Here's how the part is built. I have some questions about the finished solid (model axes, mm). A direction names the side the tool comes from. Give positions to 0.01 mm unless a question says otherwise; leave off trailing zeros. Write each loop counter-clockwise with the first axis right and the second up, starting at its lowest first coordinate (ties: lowest second). Pieces come first, ordered by that corner, then holes. Notation, with made-up numbers: (33.25, 58.25) -> (47.25, 58.25) arc R25 cw to (47.25, 88.25) -> close; hole circle Ø4 at (-34.75, 57.5). An arc over 180 degrees is marked (long way). Return JSON: item names as keys, results as strings.
from build123d import *

# Parameters (mm, degrees)
SKETCH1_W           = 19.05
SKETCH1_H           = 19.05
BOSS_EXTRUDE2_DEPTH = 6.35
SKETCH8_W           = 217.17
SKETCH8_H           = 38.1
BOSS_EXTRUDE4_DEPTH = 6.35
SKETCH8_5_W         = 217.17
SKETCH8_5_H         = 38.1
BOSS_EXTRUDE5_DEPTH = 6.4262
SKETCH9_W           = 19.05
SKETCH9_H           = 38.1
LPATTERN3_COUNT     = 11
LPATTERN3_PITCH     = 19.812
SKETCH15_R          = 12.192
BOSS_EXTRUDE6_DEPTH = 6.35
SKETCH16_W          = 38.1
SKETCH16_H          = 22.073264639
CUT_EXTRUDE1_DEPTH  = 3.302
SKETCH17_W          = 61.644203732
SKETCH17_H          = 46.422477749
CUT_EXTRUDE2_DEPTH  = 137.922
SKETCH18_W          = 24.384
SKETCH18_H          = 9.5504
BOSS_EXTRUDE7_DEPTH = 12.7


with BuildPart() as part:
    # Sketch1 → Boss-Extrude2 (new body)
    with BuildSketch(Plane(origin=(0, 0, 0), x_dir=(1, 0, 0), z_dir=(0, 1, 0))):
        with Locations((9.525, -9.525)):
            Rectangle(SKETCH1_W, SKETCH1_H)
    extrude(amount=BOSS_EXTRUDE2_DEPTH)

    # Sketch8 → Boss-Extrude4 (add)
    with BuildSketch(Plane(origin=(0, 0, 0), x_dir=(1, 0, 0), z_dir=(0, 1, 0))):
        with Locations((108.585, -9.525)):
            Rectangle(SKETCH8_W, SKETCH8_H)
    extrude(amount=BOSS_EXTRUDE4_DEPTH)

    # Sketch8<5> → Boss-Extrude5 (add)
    with BuildSketch(Plane(origin=(0, 0, 0), x_dir=(1, 0, 0), z_dir=(0, 1, 0))):
        with Locations((108.585, -9.525)):
            Rectangle(SKETCH8_5_W, SKETCH8_5_H)
    extrude(amount=-BOSS_EXTRUDE5_DEPTH)

    # Sketch9 → Loft3 section 0
    with BuildSketch(Plane(origin=(0, 6.35, 0), x_dir=(1, 0, 0), z_dir=(0, 1, 0)), mode=Mode.PRIVATE) as loft3_s0:
        with Locations((9.525, -9.525)):
            Rectangle(SKETCH9_W, SKETCH9_H)
    loft3 = loft([loft3_s0.sketch, Vertex(9.525, 26.0731, 19.05)])

    # LPattern3: Loft3 ×11
    with Locations(*[(i * LPATTERN3_PITCH, 0, 0) for i in range(1, LPATTERN3_COUNT)]):
        add(loft3)

    # Sketch15 → Boss-Extrude6 (add)
    with BuildSketch(Plane.XZ.offset(6.4262)):
        with Locations((179.07, 9.525)):
            Circle(SKETCH15_R)
        with Locations((38.1, 9.525)):
            Circle(SKETCH15_R)
        with Locations((108.585, 9.525)):
            Circle(SKETCH15_R)
    extrude(amount=BOSS_EXTRUDE6_DEPTH)

    # Sketch16 → Cut-Extrude1 (cut)
    with BuildSketch(Plane(origin=(219.71, 0, 0), x_dir=(0, 0, -1), z_dir=(1, 0, 0))):
        with Locations((-9.525, 4.61043232)):
            Rectangle(SKETCH16_W, SKETCH16_H)
    extrude(amount=-CUT_EXTRUDE1_DEPTH, mode=Mode.SUBTRACT)

    # Sketch17 → Cut-Extrude2 (cut)
    with BuildSketch(Plane.ZY):
        with Locations((9.467504242, 6.577579821)):
            Rectangle(SKETCH17_W, SKETCH17_H)
    extrude(amount=-CUT_EXTRUDE2_DEPTH, mode=Mode.SUBTRACT)

    # Sketch18 → Boss-Extrude7 (add)
    with BuildSketch(Plane.ZY.offset(-137.922)):
        with Locations((9.525, -0.0381)):
            Rectangle(SKETCH18_W, SKETCH18_H)
    extrude(amount=BOSS_EXTRUDE7_DEPTH)


solid = part.part
1. Suppose I cut it at A-A, the plane y = 10. List the corners of the cut face in (x, z) for me.
Taken from the geometry:
{"outline": "(140.45, -4.24) -> (155.97, -4.24) -> (155.97, 26.81) -> (140.45, 26.81) -> close; (160.26, -4.24) -> (175.78, -4.24) -> (175.78, 26.81) -> (160.26, 26.81) -> close; (180.07, -4.24) -> (195.6, -4.24) -> (195.6, 26.81) -> (180.07, 26.81) -> close; (199.88, -4.24) -> (215.41, -4.24) -> (215.41, 26.81) -> (199.88, 26.81) -> close"}
2. Suppose I cut it at C-C, the plane z = 3.5. List the corners of the cut face in (x, y) for me.
Taken from the geometry:
{"outline": "(125.22, -4.81) -> (137.92, -4.81) -> (137.92, -6.43) -> (168.47, -6.43) -> (168.47, -12.78) -> (189.67, -12.78) -> (189.67, -6.43) -> (216.41, -6.43) -> (216.41, 7.93) -> (212.83, 15.34) -> (202.46, 15.34) -> (198.12, 6.35) -> (197.36, 6.35) -> (193.02, 15.34) -> (182.65, 15.34) -> (178.31, 6.35) -> (177.55, 6.35) -> (173.2, 15.34) -> (162.84, 15.34) -> (158.5, 6.35) -> (157.73, 6.35) -> (153.39, 15.34) -> (143.03, 15.34) -> (138.68, 6.35) -> (137.92, 6.35) -> (137.92, 4.74) -> (125.22, 4.74) -> close"}
3. If I drill on line 1 (X direction, y = 12.5, z = 18.5); line 2 (Y direction, x = 178, z = 21); line 3 (X direction, y = 6, z = -2), over which ranges is the centre line in solid material (lowest first)? Write a range as [from, to].
Taken from the geometry:
{"line 1": "x = [141.65, 154.76], [161.47, 174.58], [181.28, 194.39], [201.09, 214.2]", "line 2": "y = [-12.78, 6.35]", "line 3": "x = [137.92, 216.41]"}
4. Suppose I cut it at B-B, the plane x = 175.5. List the corners of the cut face in (y, z) for me (3 decimals), and give its area (3 significant figures).
Taken from the geometry:
{"outline": "(-12.776, -2.133) -> (-6.426, -2.133) -> (-6.426, -9.525) -> (6.35, -9.525) -> (10.587, -3.387) -> (10.587, 26.529) -> (6.35, 28.575) -> (-6.426, 28.575) -> (-6.426, 21.183) -> (-12.776, 21.183) -> close", "area": "779 mm²"}
5. Suppose I cut it at D-D, the plane y = 23.5. List the corners of the cut face in (x, z) for me.
Taken from the geometry:
{"outline": "(146.97, 15.32) -> (149.45, 15.32) -> (149.45, 20.29) -> (146.97, 20.29) -> close; (166.78, 15.32) -> (169.26, 15.32) -> (169.26, 20.29) -> (166.78, 20.29) -> close; (186.59, 15.32) -> (189.08, 15.32) -> (189.08, 20.29) -> (186.59, 20.29) -> close; (206.4, 15.32) -> (208.89, 15.32) -> (208.89, 20.29) -> (206.4, 20.29) -> close"}
6. For pin 1 Ø4 at (x, z) = (197.5, 8.5) entering from +Y; pin 2 Ø3 at (x, z) = (201.5, -1.5) entering from -Y; pin 3 Ø5 at (y, z) = (11.5, 6) entering from +X, each with a flat end and sliding along its axis, tell me the tip position at first contact or that it passes through.
Taken from the geometry:
{"pin 1": "stops at y = 10.2", "pin 2": "stops at y = -6.43", "pin 3": "stops at x = 215.89"}
7. Which directions (+Z, -Z, +X, -X, +Y, -Y) give clear straight access to the entire face, cutting with the end or side of a thin tool? Please do faces 1 (the face through (132, 0, 21.717)), 2 (the face through (174.83, 11.97, 14.03)), 3 (the face through (132, -4.813, 9)).
Taken from the geometry:
{"face 1": "+Z, -X, +Y, -Y", "face 2": "+Z, -Z, +Y", "face 3": "+Z, -Z, -X, -Y"}
8. If we mould it in two halves opening along X, with no side actions, what happens to faces 4 (the face through (200.833, 11.967, 13.492)), 5 (the face through (177, 0, -9.525)), 6 (the face through (213.91, 13.1, 14.43))? For each: released by +X, released by -X, zero draft, split by the parting line, or undercut.
Taken from the geometry:
{"face 4": "undercut", "face 5": "zero draft", "face 6": "released by +X"}
